For this review, take the finished solid that the model builds, in its own axes (mm). A direction names the side the tool comes from. Give positions to 0.01 mm unless a question says otherwise; leave off trailing zeros. Loops run counter-clockwise (first coordinate to the right, second up) from the corner with the lowest first, then second, coordinate; pieces in that order, holes last.
```python
from build123d import *

# Parameters (mm, degrees)
SKETCH1_R               = 12.7
BOTTOM_LIP_DEPTH        = 3.302
SKETCH2_R               = 11.43
BOSS_EXTRUDE3_DEPTH     = 10.414
SKETCH3_R               = 12.192
BOSS_EXTRUDE4_DEPTH     = 1.524
SKETCH4_R               = 11.43
BOSS_EXTRUDE5_DEPTH     = 2.286
SKETCH5_R               = 12.192
BOSS_EXTRUDE7_DEPTH     = 1.524
SKETCH6_R               = 12.192
BOSS_EXTRUDE8_DEPTH     = 3.302
BOSS_EXTRUDE8_TAPER     = 42.72727272
SKETCH12_R              = 7.239
BOSS_EXTRUDE9_DEPTH     = 0.508
SKETCH13_R              = 9.14209071
CUT_EXTRUDE2_DEPTH      = 1.27
SKETCH14_R              = 7.239
BOSS_EXTRUDE10_DEPTH    = 1.778
CUT_EXTRUDE3_DEPTH      = 30.071628781
CUT_EXTRUDE3_DEPTH_BACK = 30.071628781
SKETCH15_R              = 2.794
SKETCH16_R              = 9.525
CUT_EXTRUDE4_DEPTH      = 20.32
SKETCH17_R              = 7.239
SKETCH17_R_2            = 6.35
BOSS_EXTRUDE11_DEPTH    = 2.54
SKETCH18_R              = 3.911149558
BOSS_EXTRUDE15_DEPTH    = 0.508
SKETCH19_R              = 2.794
CUT_EXTRUDE5_DEPTH      = 30.472757319
SKETCH20_R              = 0.508
BOSS_EXTRUDE16_DEPTH    = 0.508


with BuildPart() as part:
    # Sketch1 → Bottom_Lip (new body)
    with BuildSketch(Plane(origin=(0, 0, 0), x_dir=(1, 0, 0), z_dir=(0, 1, 0))):
        with Locations(Location((0, 0, 0), (0, 0, 90))):
            Circle(SKETCH1_R)
    extrude(amount=BOTTOM_LIP_DEPTH)

    # Sketch2 → Boss-Extrude3 (add)
    with BuildSketch(Plane(origin=(0, 3.302, 0), x_dir=(1, 0, 0), z_dir=(0, 1, 0))):
        with Locations(Location((0, 0, 0), (0, 0, 270))):
            Circle(SKETCH2_R)
    extrude(amount=BOSS_EXTRUDE3_DEPTH)

    # Sketch3 → Boss-Extrude4 (add)
    with BuildSketch(Plane(origin=(0, 13.716, 0), x_dir=(1, 0, 0), z_dir=(0, 1, 0))):
        with Locations(Location((0, 0, 0), (0, 0, 90))):
            Circle(SKETCH3_R)
    extrude(amount=BOSS_EXTRUDE4_DEPTH)

    # Sketch4 → Boss-Extrude5 (add)
    with BuildSketch(Plane(origin=(0, 15.24, 0), x_dir=(1, 0, 0), z_dir=(0, 1, 0))):
        with Locations(Location((0, 0, 0), (0, 0, 270))):
            Circle(SKETCH4_R)
    extrude(amount=BOSS_EXTRUDE5_DEPTH)

    # Sketch5 → Boss-Extrude7 (add)
    with BuildSketch(Plane(origin=(0, 17.526, 0), x_dir=(1, 0, 0), z_dir=(0, 1, 0))):
        with Locations(Location((0, 0, 0), (0, 0, 90))):
            Circle(SKETCH5_R)
    extrude(amount=BOSS_EXTRUDE7_DEPTH)


with BuildPart() as body_2:
    # Sketch6 → Boss-Extrude8 (new body)
    with BuildSketch(Plane(origin=(0, 19.05, 0), x_dir=(1, 0, 0), z_dir=(0, 1, 0))):
        with Locations(Location((0, 0, 0), (0, 0, 90))):
            Circle(SKETCH6_R)
    extrude(amount=BOSS_EXTRUDE8_DEPTH, taper=BOSS_EXTRUDE8_TAPER)

    # Sketch12 → Boss-Extrude9 (add)
    with BuildSketch(Plane(origin=(0, 22.352, 0), x_dir=(1, 0, 0), z_dir=(0, 1, 0))):
        with Locations(Location((0, 0, 0), (0, 0, 270))):
            Circle(SKETCH12_R)
    extrude(amount=BOSS_EXTRUDE9_DEPTH)

    # Sketch13 → Cut-Extrude2 (cut)
    with BuildSketch(Plane(origin=(0, 22.352, 0), x_dir=(1, 0, 0), z_dir=(0, 1, 0))):
        with Locations(Location((0, 0, 0), (0, 0, 270))):
            Circle(SKETCH13_R)
    extrude(amount=-CUT_EXTRUDE2_DEPTH, mode=Mode.SUBTRACT)


with BuildPart() as body_3:
    # of the pieces the cut leaves, the one that is kept (cut_extrude2_keep)
    add(body_2.part.solids().sort_by_distance((0, 19.05, -12.192))[0])

    # Sketch14 → Boss-Extrude10 (add)
    with BuildSketch(Plane(origin=(0, 21.082, 0), x_dir=(1, 0, 0), z_dir=(0, 1, 0))):
        with Locations(Location((0, 0, 0), (0, 0, 270))):
            Circle(SKETCH14_R)
    extrude(amount=BOSS_EXTRUDE10_DEPTH)

    # Sketch15 → Cut-Extrude3 (cut, two sides: drawn at the far end of the back side and taken through both)
    with BuildSketch(Plane(origin=(0, 22.86, 0), x_dir=(1, 0, 0), z_dir=(0, 1, 0)).offset(-CUT_EXTRUDE3_DEPTH_BACK)):
        with Locations(Location((0, 0, 0), (0, 0, 270))):
            Circle(SKETCH15_R)
    extrude(amount=CUT_EXTRUDE3_DEPTH + CUT_EXTRUDE3_DEPTH_BACK, mode=Mode.SUBTRACT)


with BuildPart() as cut_extrude4_tool:
    # Sketch16 → Cut-Extrude4 (new body)
    with BuildSketch(Plane.XZ):
        with Locations(Location((0, 0, 0), (0, 0, 270))):
            Circle(SKETCH16_R)
    extrude(amount=-CUT_EXTRUDE4_DEPTH)


with BuildPart() as part_1:
    add(part.part)

    # Cut-Extrude4: cut by cut_extrude4_tool
    add(cut_extrude4_tool.part, mode=Mode.SUBTRACT)



with BuildPart() as body_3_1:
    add(body_3.part)

    # Cut-Extrude4: cut by cut_extrude4_tool
    add(cut_extrude4_tool.part, mode=Mode.SUBTRACT)


with BuildPart() as part_2:
    add(part_1.part)

    add(body_3_1.part)  # Boss-Extrude11 merges body 3
    # Sketch17 → Boss-Extrude11 (add)
    with BuildSketch(Plane.XZ.offset(-20.32)):
        with Locations(Location((0, 0, 0), (0, 0, 90))):
            Circle(SKETCH17_R)
        with Locations(Location((0, 0, 0), (0, 0, 270))):
            Circle(SKETCH17_R_2, mode=Mode.SUBTRACT)
    extrude(amount=BOSS_EXTRUDE11_DEPTH)

    # Sketch18 → Boss-Extrude15 (add)
    with BuildSketch(Plane(origin=(0, 22.86, 0), x_dir=(1, 0, 0), z_dir=(0, 1, 0))):
        with Locations(Location((0, 0, 0), (0, 0, 270))):
            Circle(SKETCH18_R)
    extrude(amount=BOSS_EXTRUDE15_DEPTH)

    # Sketch19 → Cut-Extrude5 (cut, through all)
    with BuildSketch(Plane(origin=(0, 23.368, 0), x_dir=(1, 0, 0), z_dir=(0, 1, 0))):
        with Locations(Location((0, 0, 0), (0, 0, 270))):
            Circle(SKETCH19_R)
    extrude(amount=-CUT_EXTRUDE5_DEPTH, mode=Mode.SUBTRACT)

    # Sketch20 → Boss-Extrude16 (add)
    with BuildSketch(Plane(origin=(0, 22.86, 0), x_dir=(1, 0, 0), z_dir=(0, 1, 0))):
        with Locations(Location((3.942013927, -3.942013927, 0), (0, 0, 270))):
            Circle(SKETCH20_R)
        with Locations(Location((-3.942013927, -3.942013927, 0), (0, 0, 270))):
            Circle(SKETCH20_R)
        with Locations(Location((-3.942013927, 3.942013927, 0), (0, 0, 270))):
            Circle(SKETCH20_R)
        with Locations(Location((3.942013927, 3.942013927, 0), (0, 0, 270))):
            Circle(SKETCH20_R)
    extrude(amount=BOSS_EXTRUDE16_DEPTH)


solid = part_2.part
```
Q1. For probe 1 along Y at (x, z) = (4, 10.75); probe 2 along Y at (x, z) = (4.5, 3); probe 3 along Y at (x, z) = (5.5, 5.5), list the stretches that pass through material, from the lowest coordinate up.
Answers:
probe 1: y = 0 to 3.3, 13.72 to 15.24, 17.53 to 19.83
probe 2: y = 20.32 to 22.86
probe 3: y = 20.32 to 21.08
Q2. For pin 1 Ø8 at (x, z) = (-1, 9.5) entering from +Y; pin 2 Ø4 at (y, z) = (4.5, 4) entering from -X; pin 3 Ø5 at (x, z) = (8, 8) entering from +Y; pin 4 Ø4.5 at (x, z) = (0, 0) entering from -Y, all flat-tipped, find the tip position at first contact; note any pin that passes through.
Answers:
pin 1: stops at y = 22.86
pin 2: stops at x = -12.47
pin 3: stops at y = 22.35
pin 4: passes through
Q3. Machinability: for faces 4 (the cylindrical face through (3.446, 23.11, 3.832)), 5 (the flat face through (-11, 17.526, -4)), 6 (the cylindrical face through (7.7, 1.6, 10.1)), 7 (the flat face through (4, 23.368, -4)), 8 (the flat face through (7.1, 20.32, -2.1)), which of the approach directions +Z, -Z, +X, -X, +Y, -Y give a long, thin tool a straight path to every point of the face, cutting with its end or side? Answer none if there is none.
Answers:
face 4: +Y
face 5: none
face 6: +Y, -Y
face 7: +Z, -Z, +X, -X, +Y
face 8: -Y
Q4. Consider section A-A on y = 10.75. Give the boundary of the cut face in (x, z) (3 decimals).
Answers:
outline: circle Ø22.86 at (0, 0); hole circle Ø19.05 at (0, 0)
Q5. Mouldability with a two-part tool opening along Y and no side actions: class faces 1 (the cylindrical face through (-2.728, 21.865, -0.606)), 2 (the flat face through (-11, 13.716, -4)), 3 (the flat face through (-4, 23.368, -4)) as +Y half, -Y half, draft (parallel to the pull), parting line (faces both ways), or undercut.
Answers:
face 1: draft
face 2: undercut
face 3: +Y half
